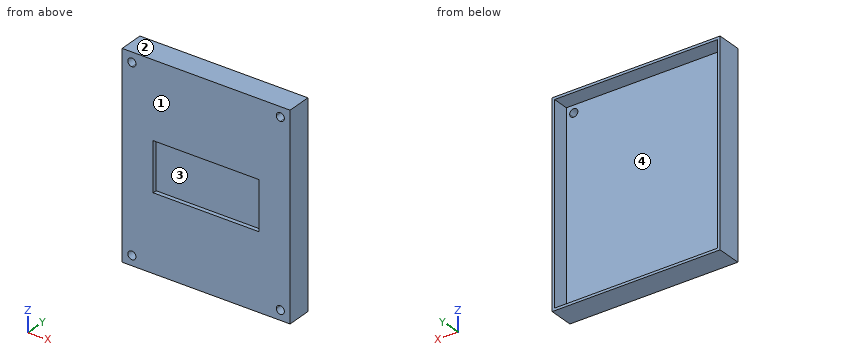
```python
from build123d import *

# Parameters (mm, degrees)
SKETCH1_W           = 206
SKETCH1_H           = 246
BOSS_EXTRUDE1_DEPTH = 60
SKETCH2_W           = 200
SKETCH2_H           = 240
CUT_EXTRUDE1_DEPTH  = 50
CUT_EXTRUDE3_DEPTH  = 172.283390905
SKETCH5_W           = 206
SKETCH5_H           = 246
CUT_EXTRUDE4_DEPTH  = 30
SKETCH6_W           = 130
SKETCH6_H           = 60
CUT_EXTRUDE5_DEPTH  = 5


with BuildPart() as part:
    # Sketch1 → Boss-Extrude1 (new body)
    with BuildSketch(Plane(origin=(0, 0, 0), x_dir=(1, 0, 0), z_dir=(0, 1, 0))):
        Rectangle(SKETCH1_W, SKETCH1_H)
    extrude(amount=BOSS_EXTRUDE1_DEPTH)

    # Sketch2 → Cut-Extrude1 (cut)
    with BuildSketch(Plane(origin=(0, 60, 0), x_dir=(1, 0, 0), z_dir=(0, 1, 0))):
        Rectangle(SKETCH2_W, SKETCH2_H)
    extrude(amount=-CUT_EXTRUDE1_DEPTH, mode=Mode.SUBTRACT)

    # Sketch3 → Cut-Extrude3 (cut, through all)
    with BuildSketch(Plane.XZ):
        with BuildLine():
            Line((-91, 106), (-91, 111))
            Line((-91, 111), (-86, 111))
            ThreePointArc((-86, 111), (-94.535533906, 114.535533906), (-91, 106))
        make_face()
        with BuildLine():
            Line((-86, 111), (-91, 111))
            Line((-91, 111), (-91, 106))
            ThreePointArc((-91, 106), (-87.464466094, 107.464466094), (-86, 111))
        make_face()
        with BuildLine():
            ThreePointArc((96, 111), (91, 116), (86, 111))
            Line((86, 111), (91, 111))
            Line((91, 111), (91, 106))
            ThreePointArc((91, 106), (94.535533906, 107.464466094), (96, 111))
        make_face()
        with BuildLine():
            Line((91, 111), (86, 111))
            ThreePointArc((86, 111), (87.464466094, 107.464466094), (91, 106))
            Line((91, 106), (91, 111))
        make_face()
        with BuildLine():
            ThreePointArc((96, -111), (94.535533906, -107.464466094), (91, -106))
            Line((91, -106), (91, -111))
            Line((91, -111), (86, -111))
            ThreePointArc((86, -111), (91, -116), (96, -111))
        make_face()
        with BuildLine():
            Line((91, -111), (91, -106))
            ThreePointArc((91, -106), (87.464466094, -107.464466094), (86, -111))
            Line((86, -111), (91, -111))
        make_face()
        with BuildLine():
            ThreePointArc((-86, -111), (-87.464466094, -107.464466094), (-91, -106))
            Line((-91, -106), (-91, -111))
            Line((-91, -111), (-86, -111))
        make_face()
        with BuildLine():
            Line((-91, -111), (-91, -106))
            ThreePointArc((-91, -106), (-94.535533906, -114.535533906), (-86, -111))
            Line((-86, -111), (-91, -111))
        make_face()
    extrude(amount=-CUT_EXTRUDE3_DEPTH, mode=Mode.SUBTRACT)

    # Sketch5 → Cut-Extrude4 (cut)
    with BuildSketch(Plane(origin=(0, 60, 0), x_dir=(1, 0, 0), z_dir=(0, 1, 0))):
        Rectangle(SKETCH5_W, SKETCH5_H)
    extrude(amount=-CUT_EXTRUDE4_DEPTH, mode=Mode.SUBTRACT)

    # Sketch6 → Cut-Extrude5 (cut)
    with BuildSketch(Plane.XZ):
        Rectangle(SKETCH6_W, SKETCH6_H)
    extrude(amount=-CUT_EXTRUDE5_DEPTH, mode=Mode.SUBTRACT)


solid = part.part
```
For this review, take the finished solid that the model builds, in its own axes (mm). Face numbers are marked on the shaded views. Round coordinates to 2 decimals unless told otherwise and drop trailing zeros. Order: outer loops, then holes, each group sorted by start corner. A loop starts at its lowest first (then second) coordinate and runs counter-clockwise, first axis right, second up.
Q1. Mouldability with a two-part tool opening along Z and no side actions: class the marked faces 1, 2, 3 and 4 as pulls with the +Z half, pulls with the -Z half, needs draft (parallel to the pull), parting line crosses it, or undercut.
Findings below:
face 1: needs draft
face 2: pulls with the +Z half
face 3: undercut
face 4: undercut
Q2. Insertion check: P1, Ø18, axis at x = -14.5, z = 3, coming from the -Y side; P2, Ø11.5, axis at x = -91, z = -111, coming from the +Y side. Each pin has a flat end and moves straight along its axis. Give the tip position at first contact, or say it passes through.
Findings below:
P1: stops at y = 5
P2: stops at y = 10
Q3. Wall thickness on line 1 (X direction, y = 3.5, z = -111); line 2 (Z direction, x = -91, y = 5); line 3 (X direction, y = 25, z = 29): over which ranges is each line inside the solid? List them lowest first.
Findings below:
line 1: x = -103 to -96, -86 to 86, 96 to 103
line 2: z = -123 to -116, -106 to 106, 116 to 123
line 3: x = -103 to -100, 100 to 103
Q4. We need section C-C, the plane z = 103. Give the boundary of the cut face in (x, y), plus the area to 3 significant figures.
Findings below:
outline: (-103, 0) - (103, 0) - (103, 30) - (100, 30) - (100, 10) - (-100, 10) - (-100, 30) - (-103, 30) - close
area: 2,180 mm2
Q5. We need section A-A, the plane y = 16.5. Give the boundary of the cut face in (x, z), plus the area to 3 significant figures.
Findings below:
outline: (-103, -123) - (103, -123) - (103, 123) - (-103, 123) - close; hole (-100, -120) - (100, -120) - (100, 120) - (-100, 120) - close
area: 2,680 mm2
Q6. We need section B-B, the plane x = -61. Give the boundary of the cut face in (y, z).
Findings below:
outline: (0, -123) - (30, -123) - (30, -120) - (10, -120) - (10, 120) - (30, 120) - (30, 123) - (0, 123) - (0, 30) - (5, 30) - (5, -30) - (0, -30) - close
